Read the model definition and answer for the solid it produces. Units are mm, in the model's axes. Face numbers are marked on the shaded views. Give positions to 0.01 mm unless a question says otherwise; leave off trailing zeros. Loops run counter-clockwise (first coordinate to the right, second up) from the corner with the lowest first, then second, coordinate; pieces in that order, holes last. Notation, with made-up numbers: (49.25, 20.25) - (56.25, 20.25) arc R22 cw to (56.25, 49.25) - close; hole circle Ø3 at (-8, 33.25). An arc over 180 degrees is marked (long way). Use a Markdown table: item, result. Add a question column.
Item 1: A cutting plane is placed at C-C (y = 6). Determine the outline of the cut face in (x, z), plus the area to 3 significant figures.
Item 2: Consider probe 1 along Z at (x, y) = (0, 6.5); probe 2 along X at (y, z) = (7.25, 1.25); probe 3 along Y at (x, z) = (3, -2.25). Determine where each line is inside the solid, lowest interval first. Write a range as [from, to].
Item 3: Each of these flat-tipped pins is pushed along its axis until it touches: P1, Ø1.5, axis at y = 9, z = -2.5, coming from the -X side; P2, Ø4, axis at y = 4.5, z = -2.5, coming from the +X side; P3, Ø1.5, axis at y = 4, z = -2, coming from the -X side. Where does it stop, or does it pass through?
Item 4: For a pull along X with two mould halves and no side action, classify the marked faces 1, 2 and 3 as +X half, -X half, draft (parallel to the pull), parting line (faces both ways), or undercut.
Item 5: A cutting plane is placed at A-A (x = 0). Determine the outline of the cut face in (y, z), plus the area to 3 significant figures.
Item 6: A cutting plane is placed at B-B (z = 0). Determine the outline of the cut face in (x, y).
Autodesk Inventor part; units mm, degrees
ref_plane "YZ Plane" through (0, 0, 0) normal (1, 0, 0) x (0, 1, 0)
ref_plane "XZ Plane" through (0, 0, 0) normal (0, 1, 0) x (-1, 0, 0)
ref_plane "XY Plane" through (0, 0, 0) normal (0, 0, 1) x (1, 0, 0)
sketch "スケッチ1" plane through (0, 0, 0) normal (0, 1, 0) x (-1, 0, 0)
  circle A0 centre (0, 0) radius 4
  dimension "d0" = 8
extrude "押し出し1" add sketch "スケッチ1" along normal blind 12
sketch "スケッチ2" plane through (0, 12, 0) normal (0, 1, 0) x (1, 0, 0)
  circle A0 centre (0, 0) radius 1.65
  dimension "d3" = 3.3
extrude "押し出し2" cut sketch "スケッチ2" against normal through all
thread "ねじ1"
fillet "フィレット1" radius 0.3 4 edges at (-1.65, 12, 0) (4, 12, 0) (-1.65, 0, 0) (4, 0, 0)
properties part number "ARL-412KE"
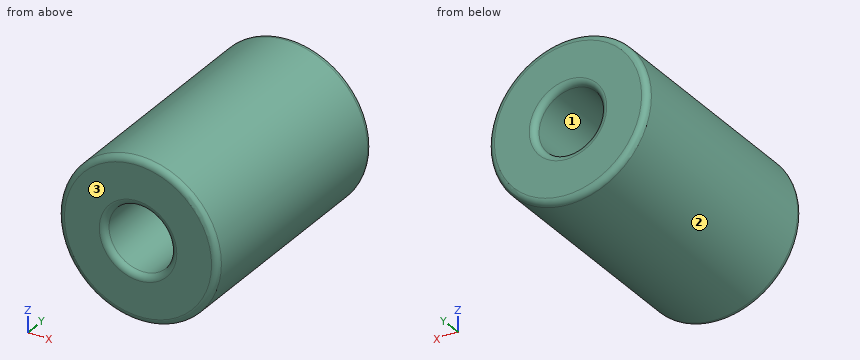
Geometry says:
| question | item | result |
|---|---|---|
| 1 | outline | circle Ø8 at (0, 0); hole circle Ø3.3 at (0, 0) |
| 1 | area | 41.7 mm² |
| 2 | probe 1 | [-4, -1.65], [1.65, 4] |
| 2 | probe 2 | [-3.8, -1.08], [1.08, 3.8] |
| 2 | probe 3 | [0, 12] |
| 3 | P1 | x = -3.6 |
| 3 | P2 | x = 3.97 |
| 3 | P3 | x = -3.8 |
| 4 | face 1 | undercut |
| 4 | face 2 | parting line |
| 4 | face 3 | draft |
| 5 | outline | (0, -3.7) arc R0.3 ccw to (0.3, -4) - (11.7, -4) arc R0.3 ccw to (12, -3.7) - (12, -1.95) arc R0.3 ccw to (11.7, -1.65) - (0.3, -1.65) arc R0.3 ccw to (0, -1.95) - close; (0, 1.95) arc R0.3 ccw to (0.3, 1.65) - (11.7, 1.65) arc R0.3 ccw to (12, 1.95) - (12, 3.7) arc R0.3 ccw to (11.7, 4) - (0.3, 4) arc R0.3 ccw to (0, 3.7) - close |
| 5 | area | 56.2 mm² |
| 6 | outline | (-4, 0.3) arc R0.3 ccw to (-3.7, 0) - (-1.95, 0) arc R0.3 ccw to (-1.65, 0.3) - (-1.65, 11.7) arc R0.3 ccw to (-1.95, 12) - (-3.7, 12) arc R0.3 ccw to (-4, 11.7) - close; (1.65, 0.3) arc R0.3 ccw to (1.95, 0) - (3.7, 0) arc R0.3 ccw to (4, 0.3) - (4, 11.7) arc R0.3 ccw to (3.7, 12) - (1.95, 12) arc R0.3 ccw to (1.65, 11.7) - close |
